CAD build for the part. Positions are in the model's coordinates, mm. A direction names the side the tool comes from. Give positions to 0.01 mm unless a question says otherwise; leave off trailing zeros. Write each loop counter-clockwise with the first axis right and the second up, starting at its lowest first coordinate (ties: lowest second). Pieces come first, ordered by that corner, then holes. Notation, with made-up numbers: (51.25, 8) -> (110.25, 8) arc R28 cw to (110.25, 45) -> close; hole circle Ø9 at (-4.5, 85). An arc over 180 degrees is marked (long way). Answer in a Markdown table with one row per item. Add a question column.
```python
from build123d import *

# Parameters (mm, degrees)
SKETCH1_W           = 56.5
SKETCH1_H           = 56.2
SKETCH1_R           = 19.25
SKETCH1_R_2         = 2.25
BOSS_EXTRUDE1_DEPTH = 3.5
SKETCH2_R           = 2
BOSS_EXTRUDE2_DEPTH = 7
BOSS_EXTRUDE3_START = 35
BOSS_EXTRUDE3_DEPTH = 7.11128839
CHAMFER1_SIZE       = 2


with BuildPart() as part:
    # Sketch1 → Boss-Extrude1 (new, symmetric)
    with BuildSketch(Plane(origin=(0, 0, 0), x_dir=(0, 0, -1), z_dir=(1, 0, 0))):
        with Locations((0.36128839, 0)):
            Rectangle(SKETCH1_W, SKETCH1_H)
        with Locations((0.36128839, 0)):
            Circle(SKETCH1_R, mode=Mode.SUBTRACT)
        with Locations((-23.468210136, 23.829498526)):
            Circle(SKETCH1_R_2, mode=Mode.SUBTRACT)
        with Locations(Location((24.190786916, 23.829498526, 0), (0, 0, 180))):
            Circle(SKETCH1_R_2, mode=Mode.SUBTRACT)
        with Locations((24.190786916, -23.829498526)):
            Circle(SKETCH1_R_2, mode=Mode.SUBTRACT)
        with Locations(Location((-23.468210136, -23.829498526, 0), (0, 0, 180))):
            Circle(SKETCH1_R_2, mode=Mode.SUBTRACT)
    extrude(amount=BOSS_EXTRUDE1_DEPTH, both=True)

    # Sketch2 → Boss-Extrude2 (add)
    with BuildSketch(Plane.XZ.offset(28.1)):
        with BuildLine():
            Line((-51.5, 35), (8.5, 35))
            ThreePointArc((8.5, 35), (12.035533906, 33.535533906), (13.5, 30))
            Line((13.5, 30), (13.5, -30))
            ThreePointArc((13.5, -30), (12.035533906, -33.535533906), (8.5, -35))
            Line((8.5, -35), (-51.5, -35))
            ThreePointArc((-51.5, -35), (-55.035533906, -33.535533906), (-56.5, -30))
            Line((-56.5, -30), (-56.5, 30))
            ThreePointArc((-56.5, 30), (-55.035533906, 33.535533906), (-51.5, 35))
        make_face()
        with Locations(Location((8.5, 30, 0), (0, 0, 270))):
            Circle(SKETCH2_R, mode=Mode.SUBTRACT)
        with Locations(Location((8.5, -30, 0), (0, 0, 90))):
            Circle(SKETCH2_R, mode=Mode.SUBTRACT)
        with Locations(Location((-51.5, 30, 0), (0, 0, 90))):
            Circle(SKETCH2_R, mode=Mode.SUBTRACT)
        with Locations(Location((-51.5, -30, 0), (0, 0, 270))):
            Circle(SKETCH2_R, mode=Mode.SUBTRACT)
    extrude(amount=BOSS_EXTRUDE2_DEPTH)

    # Sketch4 → Boss-Extrude3 (add)
    with BuildSketch(Plane.XY.offset(BOSS_EXTRUDE3_START)):
        Polygon((-41.5, -28.1), (-3.5, 28.1), (3.5, 28.1), (3.5, -28.1), align=None)
    extrude(amount=-BOSS_EXTRUDE3_DEPTH)

    # Chamfer1
    chamfer1_edges = [part.edges().sort_by_distance(p)[0] for p in [
        (3.5, 23.829498526, 25.718210136),
        (3.5, 23.829498526, -26.440786916),
        (3.5, -23.829498526, -21.940786916),
        (3.5, -23.829498526, 21.218210136),
    ]]
    chamfer(chamfer1_edges, length=CHAMFER1_SIZE)


solid = part.part
```
Item 1: Slice it at D-D, the plane y = -3. List the corners of the cut face in (x, z).
Item 2: Mould opens along Y. For faces 1 (the face through (-1.035, 25.826, -23.153)), 2 (the face through (12.07, -31.55, -33.5)), 3 (the face through (-21, -28.1, 0)) say: released by +Y, released by -Y, zero draft, split by the parting line, or undercut.
Item 3: Slice it at A-A, the plane z = 12.5. List the corners of the cut face in (x, y).
Item 4: Slice it at B-B, the plane y = 12.5. List the corners of the cut face in (x, z), then the cut area to 3 significant figures.
Item 5: Drop flat-ended pins along their axis: pin 1 Ø7.5 at (x, y) = (0, -11) entering from -Z; pin 2 Ø12 at (x, z) = (-41, 3.5) entering from +Y; pin 3 Ø6 at (y, z) = (-23.83, 23.47) entering from -X. Give the stop position or say it passes through.
Item 6: Slice it at C-C, the plane z = -7.5. List the corners of the cut face in (x, y), then the cut area to 3 significant figures.
Item 7: Probe L1, parallel to X at y = -31.5, z = 30; L2, parallel to Z at x = -51, y = -31; L3, parallel to Y at x = -42, z = -13. List the from-to ranges inside material, lowest first. Write a range as from..to.
Item 8: Which spindle directions (+Z, -Z, +X, -X, +Y, -Y) get a long thin tool onto all of the face, cutting with end or side? Do faces 4 (the face through (-0.049, -11.713, 14.915)), 5 (the face through (3.5, 7, 18)), 6 (the face through (-3.5, 19, 6)). Say none if no direction does.
Answer key:
| question | item | result |
|---|---|---|
| 1 | outline | (-24.53, 27.89) -> (-3.5, 27.89) -> (-3.5, 18.65) -> (3.5, 18.65) -> (3.5, 35) -> (-24.53, 35) -> close; (-3.5, -28.61) -> (3.5, -28.61) -> (3.5, -19.38) -> (-3.5, -19.38) -> close |
| 2 | face 1 | undercut |
| 2 | face 2 | zero draft |
| 2 | face 3 | released by +Y |
| 3 | outline | (-56.5, -35.1) -> (13.5, -35.1) -> (13.5, -28.1) -> (3.5, -28.1) -> (3.5, -14.32) -> (-3.5, -14.32) -> (-3.5, -28.1) -> (-56.5, -28.1) -> close; (-3.5, 14.32) -> (3.5, 14.32) -> (3.5, 28.1) -> (-3.5, 28.1) -> close |
| 4 | outline | (-14.05, 27.89) -> (-3.5, 27.89) -> (-3.5, 14.28) -> (3.5, 14.28) -> (3.5, 35) -> (-14.05, 35) -> close; (-3.5, -28.61) -> (3.5, -28.61) -> (3.5, -15) -> (-3.5, -15) -> close |
| 4 | area | 315 mm² |
| 5 | pin 1 | stops at z = -28.61 |
| 5 | pin 2 | stops at y = -28.1 |
| 5 | pin 3 | stops at x = -3.5 |
| 6 | outline | (-56.5, -35.1) -> (13.5, -35.1) -> (13.5, -28.1) -> (3.5, -28.1) -> (3.5, -17.88) -> (-3.5, -17.88) -> (-3.5, -28.1) -> (-56.5, -28.1) -> close; (-3.5, 17.88) -> (3.5, 17.88) -> (3.5, 28.1) -> (-3.5, 28.1) -> close |
| 6 | area | 633 mm² |
| 7 | L1 | x = -56.5..-53.5, -49.5..6.5, 10.5..13.5 |
| 7 | L2 | z = -35..-31.94, -28.06..28.06, 31.94..35 |
| 7 | L3 | y = -35.1..-28.1 |
| 8 | face 4 | +X, -X |
| 8 | face 5 | +Z, -Z, +X, +Y |
| 8 | face 6 | -Z, -X, +Y |
